For this review, take the finished solid that the model builds, in its own axes (mm). Give positions to 0.01 mm unless a question says otherwise; leave off trailing zeros. Loops run counter-clockwise (first coordinate to the right, second up) from the corner with the lowest first, then second, coordinate; pieces in that order, holes last.
```python
from build123d import *

# Parameters (mm, degrees)
F1_DEPTH = 17
F2_ANGLE = 180


with BuildPart() as f1:
    # F0 (on Top) → F1 (new body)
    with BuildSketch(Plane.XY):
        Polygon((-256.887055, -71.171104), (-231.887055, -166.171104), (-201.887055, -191.171104), (-141.887055, -191.171104), (-111.887055, -166.171104), (-86.887055, -71.171104), (-121.887055, -19.446782), (-221.887055, -19.446782), align=None)
    extrude(amount=F1_DEPTH)


with BuildPart() as f1_1:
    # F2: moved
    add(f1.part.rotate(Axis((-141.887055, -191.171104, 8.5), (0, 0, 1)), F2_ANGLE))


solid = f1_1.part
```
Q1. For probe 1 along X at (y, z) = (-228, 14.75); probe 2 along X at (y, z) = (-296.5, 12.5); probe 3 along Y at (x, z) = (-78, 9.5), list the stretches that pass through material, from the lowest coordinate up.
Answers:
probe 1: x = -175 to -48.77
probe 2: x = -193.03 to -30.75
probe 3: y = -362.9 to -194.41
Q2. Consider section B-B on y = -288. Give the boundary of the cut face in (x, z), plus the area to 3 significant figures.
Answers:
outline: (-190.79, 0) - (-32.98, 0) - (-32.98, 17) - (-190.79, 17) - close
area: 2,680 mm2
Q3. Consider section C-C on x = -41. Give the boundary of the cut face in (y, z), plus the area to 3 significant figures.
Answers:
outline: (-332.03, 0) - (-257.54, 0) - (-257.54, 17) - (-332.03, 17) - close
area: 1,270 mm2
Q4. For pin 1 Ø5 at (y, z) = (-268, 4) entering from -X; pin 2 Ø2 at (x, z) = (-78, 6) entering from +Y; pin 3 Ø6 at (y, z) = (-270.5, 5.5) entering from +X, all flat-tipped, find the tip position at first contact; note any pin that passes through.
Answers:
pin 1: stops at x = -186.18
pin 2: stops at y = -193.58
pin 3: stops at x = -36.8
Q5. Consider section A-A on z = 6.75. Give the boundary of the cut face in (x, y).
Answers:
outline: (-196.89, -311.17) - (-161.89, -362.9) - (-61.89, -362.9) - (-26.89, -311.17) - (-51.89, -216.17) - (-81.89, -191.17) - (-141.89, -191.17) - (-171.89, -216.17) - close
